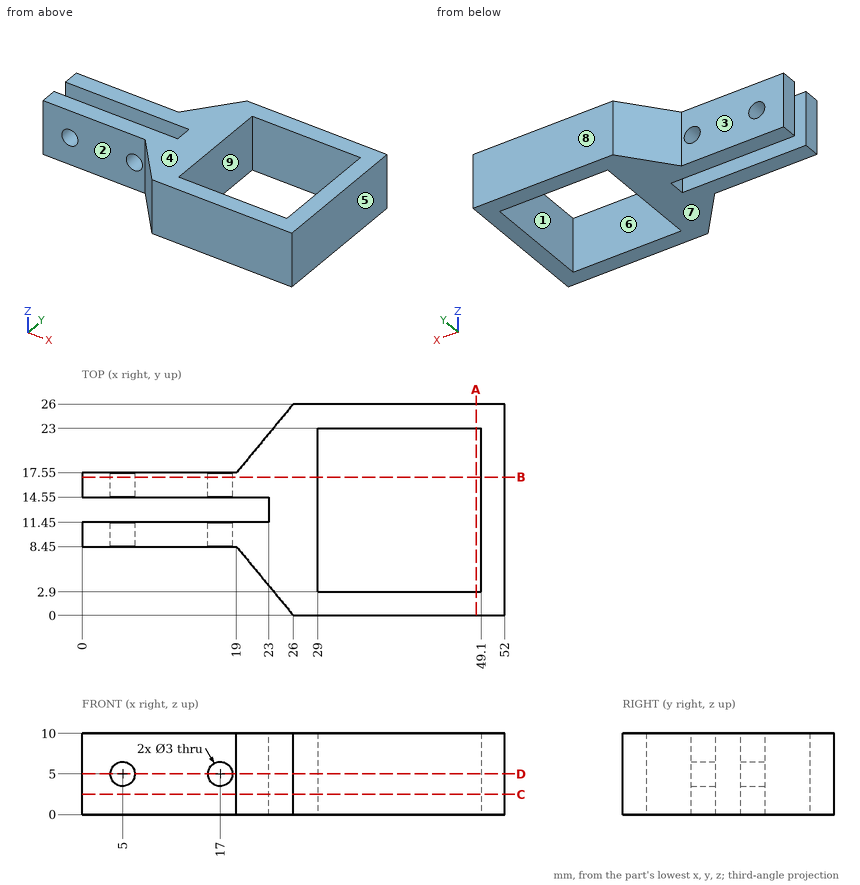
Check sheet for the drawn part. Datum: minimum x, y, z corner. Units: mm. A direction names the side the tool comes from. Give positions to 0.01 mm unless a question says otherwise; leave off trailing zeros. Order: outer loops, then holes, each group sorted by start corner. A loop starts at its lowest first (then second) coordinate and runs counter-clockwise, first axis right, second up.
1. Sectioned sample at B-B (y = 17). Record the boundary of the cut face in (x, z), then the cut area to 3 significant figures.
Completed:
outline: (0, 0) - (29, 0) - (29, 10) - (0, 10) - close; (49.1, 0) - (52, 0) - (52, 10) - (49.1, 10) - close; hole circle Ø3 at (5, 5); hole circle Ø3 at (17, 5)
area: 305 mm2
2. Access from +Z, -Z, +X, -X, +Y, -Y to the whole of each face (thin tool, end or side, straight path). Record for the marked faces 1, 2, 3, 4 and 5.
Completed:
face 1: +Z, -Z
face 2: +Z, -Z, -X, -Y
face 3: +Z, -Z, -X, +Y
face 4: +Z, +X, -X, +Y, -Y
face 5: +Z, -Z, +X, +Y, -Y
3. Scan lines: line 1 (X direction, y = 9.25, z = 5); line 2 (Y direction, x = 16, z = 8.5); line 3 (Z direction, x = 5, y = 15.7). Record each from-to range of solid material in increasing order.
Completed:
line 1: x = 0 to 3.5, 6.5 to 15.5, 18.5 to 29, 49.1 to 52
line 2: y = 8.45 to 11.45, 14.55 to 17.55
line 3: z = 0 to 3.5, 6.5 to 10
4. Sectioned sample at D-D (z = 5). State how many separate pieces and enclosed holes the cut face has, then the cut area to 3 significant figures.
Completed:
separate pieces: 5
enclosed holes: 1
area: 460 mm2
5. Depth check by flat-ended pin: pin 1 (4 mm diameter, centred on x = 5, z = 5, fed in from -Y); pin 2 (3.5 mm diameter, centred on x = 17, z = 5, fed in from +Y); pin 3 (5 mm diameter, centred on y = 22.5, z = 2, fed in from -X). Enter the tip coordinate at first touch or a pass-through.
Completed:
pin 1: stops at y = 8.45
pin 2: stops at y = 17.55
pin 3: stops at x = 21.03
6. Sectioned sample at A-A (x = 48.5). Record the boundary of the cut face in (y, z), then the cut area to 3 significant figures.
Completed:
outline: (0, 0) - (2.9, 0) - (2.9, 10) - (0, 10) - close; (23, 0) - (26, 0) - (26, 10) - (23, 10) - close
area: 59.0 mm2
7. Sectioned sample at C-C (z = 2.5). Record the boundary of the cut face in (x, y).
Completed:
outline: (0, 8.45) - (19, 8.45) - (26, 0) - (52, 0) - (52, 26) - (26, 26) - (19, 17.55) - (0, 17.55) - (0, 14.55) - (23, 14.55) - (23, 11.45) - (0, 11.45) - close; hole (29, 2.9) - (49.1, 2.9) - (49.1, 23) - (29, 23) - close
8. Draft check along Y on the marked faces 6, 7, 8 and 9. Enter one of: pulls with the +Y half, pulls with the -Y half, needs draft (parallel to the pull), parting line crosses it, or undercut.
Completed:
face 6: undercut
face 7: needs draft
face 8: pulls with the +Y half
face 9: undercut
